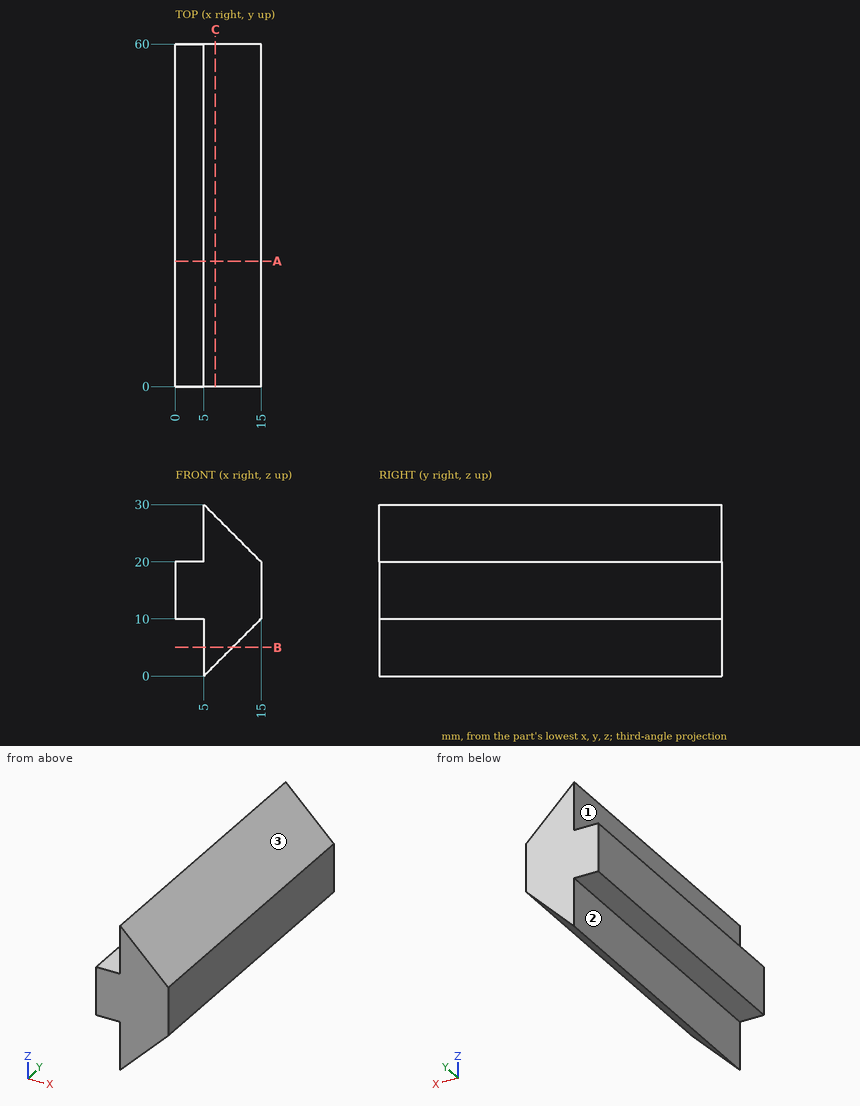
Source: three-view drawing plus pictorial views. Frame: mm from the lowest corner of the part. A direction names the side the tool comes from. Round coordinates to 2 decimals unless told otherwise and drop trailing zeros. Write each loop counter-clockwise with the first axis right and the second up, starting at its lowest first coordinate (ties: lowest second). Pieces come first, ordered by that corner, then holes. Notation, with made-up numbers: M 63.25,-27.5 L 104.25,-27.5 A22 cw 104.25,-11.5 Z; hole C 53,18 d3. An arc over 180 degrees is marked long. Write each question's results on one line, items separated by ' | '.
Q1. Section query A-A (y = 22). Return loops of the section in (x, z), and give its area (3 significant figures).
Results:
outline: M 0,10 L 5,10 L 5,0 L 15,10 L 15,20 L 5,30 L 5,20 L 0,20 Z | area: 250 mm^2
Q2. Section query C-C (x = 7). Return loops of the section in (y, z), and give its area (3 significant figures).
Results:
outline: M 0,2 L 60,2 L 60,28 L 0,28 Z | area: 1,560 mm^2
Q3. Pin query (flat end, axial travel): P1, Ø3, axis at y = 22.5, z = 5, coming from the -X side; P2, Ø1, axis at x = 7, y = 22, coming from the +Z side; P3, Ø2.5, axis at x = 2, y = 21.5, coming from the +Z side. Return the tip coordinate at first contact, or that it passes through.
Results:
P1: stops at x = 5 | P2: stops at z = 28.5 | P3: stops at z = 20
Q4. Line query: line 1 along Z through (x, y) = (2, 50); line 2 along X through (y, z) = (51, 5); line 3 along X through (y, z) = (33, 8.75). Output: solid intervals per line, ascending.
Results:
line 1: z = 10 to 20 | line 2: x = 5 to 10 | line 3: x = 5 to 13.75
Q5. Section query B-B (z = 5). Return loops of the section in (x, y).
Results:
outline: M 5,0 L 10,0 L 10,60 L 5,60 Z
Q6. Access query for the marked faces 1, 2 and 3. Directions: +Z, -Z, +X, -X, +Y, -Y. A direction counts if a zero-diameter tool reaches every point of the face in a straight line with its end or side. Return the directions, or none.
Results:
face 1: +Z, -X, +Y, -Y | face 2: -Z, -X, +Y, -Y | face 3: +Z, +X, +Y, -Y
